The model under review builds one solid part; all positions refer to its coordinate system, in mm. Round coordinates to 2 decimals unless told otherwise and drop trailing zeros. Write each loop counter-clockwise with the first axis right and the second up, starting at its lowest first coordinate (ties: lowest second). Pieces come first, ordered by that corner, then holes. Notation, with made-up numbers: (11.25, 7.25) -> (69.25, 7.25) arc R31 ccw to (69.25, 36.25) -> close; hole circle Ø8 at (43, -38.5). An arc over 180 degrees is marked (long way). Return JSON: item names as keys, results as strings. Group by question number.
1. For line 1 along X through (y, z) = (6.5, -7.75); line 2 along Z through (x, y) = (6, 5.5); line 3 along Z through (x, y) = (6, 3.25), list the stretches that pass through material, from the lowest coordinate up. Write a range as from..to.
2. Take a section at A-A, the plane x = 7.5. Write out the cut boundary in (y, z), then the cut area to 3 significant figures.
3. Take a section at C-C, the plane y = 2.75. Write out the cut boundary in (x, z).
4. Mouldability with a two-part tool opening along Z and no side actions: class faces 1 (the cylindrical face through (8.176, 4.451, -29.104)), 2 (the cylindrical face through (14.699, 4.042, -0.285)), 3 (the cylindrical face through (14.715, 7.699, -19.759)) as pulls with the +Z half, pulls with the -Z half, needs draft (parallel to the pull), parting line crosses it, or undercut.
5. Take a section at D-D, the plane x = 3.5. Write out the cut boundary in (y, z), then the cut area to 3 significant figures.
6. Take a section at B-B, the plane z = -7.75. Write out the cut boundary in (x, y), then the cut area to 3 significant figures.
7. Clearance check with a flat-ended pin moving along its axis: P1, Ø2.5, axis at x = 7.5, z = -7.75, coming from the +Y side (3 decimals). State where the tip first meets the part, or that it passes through.
from build123d import *

# Parameters (mm, degrees)
SKETCH1_W           = 15
SKETCH1_H           = 39
SKETCH1_R           = 2.25
BOSS_EXTRUDE1_DEPTH = 8
FILLET2_R           = 1
CUT_EXTRUDE1_REACH  = 44.544


with BuildPart() as part:
    # Sketch1 → Boss-Extrude1 (new body)
    with BuildSketch(Plane(origin=(0, 0, 0), x_dir=(1, 0, 0), z_dir=(0, 1, 0))):
        with Locations((7.5, 19.5)):
            Rectangle(SKETCH1_W, SKETCH1_H)
        with Locations(Location((7.5, 31.25, 0), (0, 0, 270))):
            Circle(SKETCH1_R, mode=Mode.SUBTRACT)
        with Locations(Location((7.5, 7.75, 0), (0, 0, 90))):
            Circle(SKETCH1_R, mode=Mode.SUBTRACT)
    extrude(amount=BOSS_EXTRUDE1_DEPTH)

    # Fillet2
    fillet2_edges = [part.edges().sort_by_distance(p)[0] for p in [
        (15, 8, -19.5),
        (7.5, 8, -39),
        (0, 8, -19.5),
        (7.5, 8, 0),
        (0, 4, -39),
        (15, 4, -39),
        (15, 4, 0),
        (0, 4, 0),
    ]]
    fillet(fillet2_edges, radius=FILLET2_R)

    # Cut-Extrude1: up to this face of the body (flat: up to its plane)
    cut_extrude1_end = Plane(part.part.faces().sort_by_distance((15, 3.5, -19.5))[0])
    # Sketch2 → Cut-Extrude1 (cut, up to the picked face)
    with BuildSketch(Plane.ZY, mode=Mode.PRIVATE) as cut_extrude1_sk1:
        with BuildLine():
            Line((-23.372983346, 1), (-45.302397196, 1))
            Line((-45.302397196, 1), (-45.302397196, -1))
            Line((-45.302397196, -1), (4.697602804, -1))
            Line((4.697602804, -1), (4.697602804, 1))
            Line((4.697602804, 1), (-15.627016654, 1))
            ThreePointArc((-15.627016654, 1), (-19.5, 4), (-23.372983346, 1))
        make_face()
    cut_extrude1_tool1 = split(extrude(cut_extrude1_sk1.sketch, amount=-CUT_EXTRUDE1_REACH, mode=Mode.PRIVATE), bisect_by=cut_extrude1_end, keep=Keep.BOTH, mode=Mode.PRIVATE)
    add(cut_extrude1_tool1.solids().sort_by(Axis((0, 0.330412, -20.184541), (1, 0, 0)))[0], mode=Mode.SUBTRACT)


solid = part.part
Output:
{
 "1": {"line 1": "x = 0..5.25, 9.75..15", "line 2": "z = -39..-32.93, -29.57..-9.43, -6.07..0", "line 3": "z = -39..-32.93, -29.57..-21.83, -17.17..-9.43, -6.07..0"},
 "2": {"outline": "(1, -39) -> (7, -39) arc R1 ccw to (8, -38) -> (8, -33.5) -> (1, -33.5) -> close; (1, -29) -> (8, -29) -> (8, -10) -> (1, -10) -> (1, -15.63) arc R4 cw to (1, -23.37) -> close; (1, -5.5) -> (8, -5.5) -> (8, -1) arc R1 ccw to (7, 0) -> (1, 0) -> close", "area": "192 mm^2"},
 "3": {"outline": "(0, -38) arc R1 ccw to (1, -39) -> (14, -39) arc R1 ccw to (15, -38) -> (15, -22.4) -> (0, -22.4) -> close; (0, -16.6) -> (15, -16.6) -> (15, -1) arc R1 ccw to (14, 0) -> (1, 0) arc R1 ccw to (0, -1) -> close; hole circle Ø4.5 at (7.5, -31.25); hole circle Ø4.5 at (7.5, -7.75)"},
 "4": {"face 1": "undercut", "face 2": "pulls with the +Z half", "face 3": "needs draft"},
 "5": {"outline": "(1, -39) -> (7, -39) arc R1 ccw to (8, -38) -> (8, -1) arc R1 ccw to (7, 0) -> (1, 0) -> (1, -15.63) arc R4 cw to (1, -23.37) -> close", "area": "255 mm^2"},
 "6": {"outline": "(0, 1) -> (5.25, 1) -> (5.25, 8) -> (1, 8) arc R1 ccw to (0, 7) -> close; (9.75, 1) -> (15, 1) -> (15, 7) arc R1 ccw to (14, 8) -> (9.75, 8) -> close", "area": "73.1 mm^2"},
 "7": {"P1": "passes through"}
}
